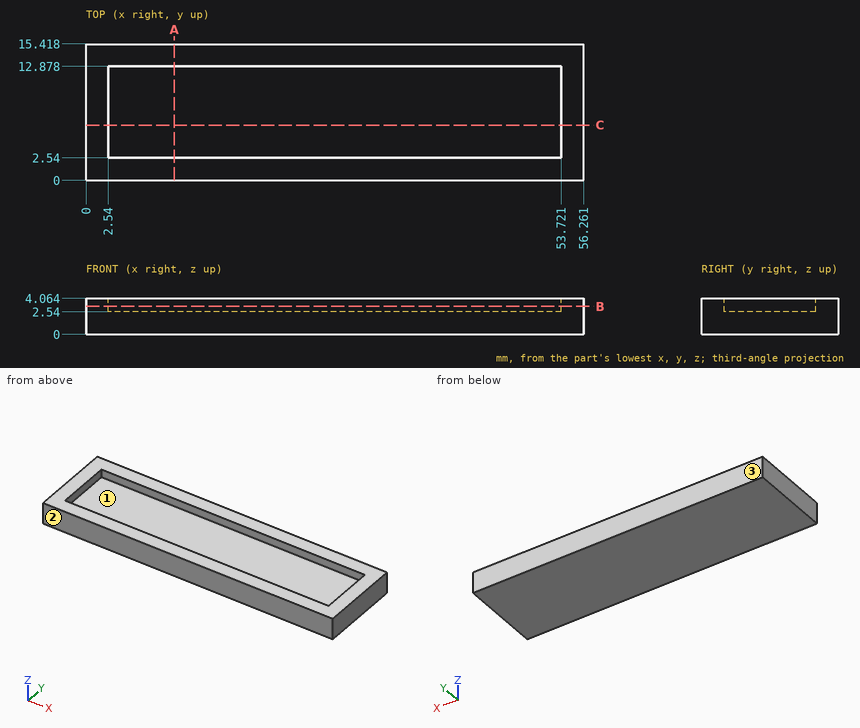
For this review, use the dimensioned drawing (mm, ordinates from the lowest corner) and the shaded views. Give positions to 0.01 mm unless a question says otherwise; leave off trailing zeros. Order: outer loops, then holes, each group sorted by start corner. A loop starts at its lowest first (then second) coordinate and runs counter-clockwise, first axis right, second up. Notation, with made-up numbers: M 41.25,-21 L 46.25,-21 A22 ccw 46.25,16 Z; hole C 10,-23 d2. An arc over 180 degrees is marked long. Use one line per item in the form item = value. Start each with the question number.
Item 1: We need section A-A on x = 10. Give the boundary of the cut face in (y, z).
Item 2: The part is to be moulded in two halves that separate along Y. For the marked faces 1, 2 and 3, say which applies: pulls with the +Y half, pulls with the -Y half, needs draft (parallel to the pull), parting line crosses it, or undercut.
Item 3: Insertion check: pin 1 Ø1.5 at (x, z) = (19.5, 3) entering from -Y. The pin has a flat end and moves straight along its axis. Give the tip position at first contact, or say it passes through.
Item 4: We need section C-C on y = 6.25. Give the boundary of the cut face in (x, z), plus the area to 3 significant figures.
Item 5: We need section B-B on z = 3.15. Give the boundary of the cut face in (x, y), plus the area to 3 significant figures.
Item 6: To check wall thickness, follow line 1 along Y through (x, z) = (28, 3.45); line 2 along X through (y, z) = (12, 3.8); line 3 along Z through (x, y) = (6, 6.75). State the ranges of each line that lie inside material, in increasing order. Write a range as from..to.
Completed:
q1.outline = M 0,0 L 15.42,0 L 15.42,4.06 L 12.88,4.06 L 12.88,2.54 L 2.54,2.54 L 2.54,4.06 L 0,4.06 Z
q2.face_1 = undercut
q2.face_2 = pulls with the -Y half
q2.face_3 = pulls with the +Y half
q3.pin_1 = 0
q4.outline = M 0,0 L 56.26,0 L 56.26,4.06 L 53.72,4.06 L 53.72,2.54 L 2.54,2.54 L 2.54,4.06 L 0,4.06 Z
q4.area = 151 mm²
q5.outline = M 0,0 L 56.26,0 L 56.26,15.42 L 0,15.42 Z; hole M 2.54,2.54 L 53.72,2.54 L 53.72,12.88 L 2.54,12.88 Z
q5.area = 338 mm²
q6.line_1 = 0..2.54, 12.88..15.42
q6.line_2 = 0..2.54, 53.72..56.26
q6.line_3 = 0..2.54
